from build123d import *

# Parameters (mm, degrees)
SKETCH1_W           = 25.4
SKETCH1_H           = 25.4
BOSS_EXTRUDE2_DEPTH = 254
SKETCH2_W           = 20.302766191
SKETCH2_H           = 19.05
CUT_EXTRUDE1_DEPTH  = 257.527425434
CUT_EXTRUDE2_DEPTH  = 257.527425434
SKETCH6_R           = 3.175
CUT_EXTRUDE5_DEPTH  = 257.527425553
SKETCH4_R           = 3.175
CUT_EXTRUDE6_DEPTH  = 257.527425553
SKETCH7_R           = 3.175
CUT_EXTRUDE7_DEPTH  = 257.527425553


with BuildPart() as part:
    # Sketch1 → Boss-Extrude2 (new body)
    with BuildSketch(Plane.XY):
        with Locations((12.7, 12.7)):
            Rectangle(SKETCH1_W, SKETCH1_H)
    extrude(amount=BOSS_EXTRUDE2_DEPTH)

    # Sketch2 → Cut-Extrude1 (cut, through all)
    with BuildSketch(Plane(origin=(0, 0, 0), x_dir=(-1, 0, 0), z_dir=(0, 0, -1))):
        with Locations((-13.326383096, 12.7)):
            Rectangle(SKETCH2_W, SKETCH2_H)
    extrude(amount=-CUT_EXTRUDE1_DEPTH, mode=Mode.SUBTRACT)

    # Sketch3 → Cut-Extrude2 (cut, through all)
    with BuildSketch(Plane(origin=(0, 25.4, 0), x_dir=(1, 0, 0), z_dir=(0, 1, 0))):
        with BuildLine():
            add(Edge.make_bspline(
                [(12.7, 0), (0, 0), (0, -30.465860076)],
                knots=[6.283185307, 6.283185307, 6.283185307, 7.853981634, 7.853981634, 7.853981634], degree=2, weights=[1, 0.707106781, 1]))
            Line((12.7, 0), (0, 0))
            Line((0, 0), (0, -30.465860076))
        make_face()
        with BuildLine():
            Line((25.4, 0), (12.7, 0))
            add(Edge.make_bspline(
                [(25.4, -30.465860076), (25.4, 0), (12.7, 0)],
                knots=[4.71238898, 4.71238898, 4.71238898, 6.283185307, 6.283185307, 6.283185307], degree=2, weights=[1, 0.707106781, 1]))
            Line((25.4, -30.465860076), (25.4, 0))
        make_face()
    extrude(amount=-CUT_EXTRUDE2_DEPTH, mode=Mode.SUBTRACT)

    # Sketch6 → Cut-Extrude5 (cut, through all)
    with BuildSketch(Plane(origin=(0, 25.4, 0), x_dir=(1, 0, 0), z_dir=(0, 1, 0))):
        with Locations(Location((12.7, -12.7, 0), (0, 0, 270))):
            Circle(SKETCH6_R)
    extrude(amount=-CUT_EXTRUDE5_DEPTH, mode=Mode.SUBTRACT)

    # Sketch4 → Cut-Extrude6 (cut, through all)
    with BuildSketch(Plane(origin=(0, 25.4, 0), x_dir=(1, 0, 0), z_dir=(0, 1, 0))):
        with Locations(Location((12.7, -101.6, 0), (0, 0, 270))):
            Circle(SKETCH4_R)
    extrude(amount=-CUT_EXTRUDE6_DEPTH, mode=Mode.SUBTRACT)

    # Sketch7 → Cut-Extrude7 (cut, through all)
    with BuildSketch(Plane(origin=(0, 25.4, 0), x_dir=(1, 0, 0), z_dir=(0, 1, 0))):
        with Locations(Location((12.7, -241.3, 0), (0, 0, 270))):
            Circle(SKETCH7_R)
    extrude(amount=-CUT_EXTRUDE7_DEPTH, mode=Mode.SUBTRACT)


solid = part.part
Geometry check sheet. Reference: the model listing, model coordinates, mm. A direction names the side the tool comes from. Give positions to 0.01 mm unless a question says otherwise; leave off trailing zeros. Loops run counter-clockwise (first coordinate to the right, second up) from the corner with the lowest first, then second, coordinate; pieces in that order, holes last. Notation, with made-up numbers: (22.5, -32.5) -> (63.5, -32.5) arc R15 ccw to (63.5, -12.5) -> close; hole circle Ø2 at (55, 6.25). An arc over 180 degrees is marked (long way). Answer in a Markdown table with one row per item. Add a question column.
1) Cross-section at B-B on z = 208.5. Record the boundary of the cut face in (x, y) (3 decimals), and give its area (3 significant figures).
2) Cross-section at A-A on z = 241.3. Record the boundary of the cut face in (x, y) (3 decimals).
3) Material ranges on probe 1 along Y at (x, z) = (21.25, 178) (3 decimals); probe 2 along X at (y, z) = (11, 57) (3 decimals); probe 3 along X at (y, z) = (24.5, 101.6) (3 decimals), recorded low to high. Write a range as from..to.
4) Cross-section at C-C on z = 101. Record the boundary of the cut face in (x, y) (3 decimals), and give its area (3 significant figures).
5) Set-up check for faces 1 (the face through (3.175, 13, 130)), 2 (the face through (10.77, 1.61, 10.18)): record each of +Z, -Z, +X, -X, +Y, -Y from which the full face is reachable in a straight line by a thin tool's end or side.
6) Draft check along X on faces 3 (the face through (13, 25.4, 125)), 4 (the face through (23.478, 13, 132)), 5 (the face through (25.4, 13, 141)). Enter one of: pulls with the +X half, pulls with the -X half, needs draft (parallel to the pull), parting line crosses it, or undercut.
7) Gauge pin test, flat end, axial feed: P1, Ø5, axis at x = 12.7, z = 12.7, coming from the -Y side. Record the tip position at first contact, or that the pin passes through.
Outcome:
| question | item | result |
|---|---|---|
| 1 | outline | (0, 0) -> (25.4, 0) -> (25.4, 25.4) -> (0, 25.4) -> close; hole (3.175, 3.175) -> (23.478, 3.175) -> (23.478, 22.225) -> (3.175, 22.225) -> close |
| 1 | area | 258 mm^2 |
| 2 | outline | (0, 0) -> (9.525, 0) -> (9.525, 3.175) -> (3.175, 3.175) -> (3.175, 22.225) -> (9.525, 22.225) -> (9.525, 25.4) -> (0, 25.4) -> close; (15.875, 0) -> (25.4, 0) -> (25.4, 25.4) -> (15.875, 25.4) -> (15.875, 22.225) -> (23.478, 22.225) -> (23.478, 3.175) -> (15.875, 3.175) -> close |
| 3 | probe 1 | y = 0..3.175, 22.225..25.4 |
| 3 | probe 2 | x = 0..3.175, 23.478..25.4 |
| 3 | probe 3 | x = 0..9.525, 15.875..25.4 |
| 4 | outline | (0, 0) -> (9.582, 0) -> (9.582, 3.175) -> (3.175, 3.175) -> (3.175, 22.225) -> (9.582, 22.225) -> (9.582, 25.4) -> (0, 25.4) -> close; (15.818, 0) -> (25.4, 0) -> (25.4, 25.4) -> (15.818, 25.4) -> (15.818, 22.225) -> (23.478, 22.225) -> (23.478, 3.175) -> (15.818, 3.175) -> close |
| 4 | area | 219 mm^2 |
| 5 | face 1 | +Z, -Z |
| 5 | face 2 | +Y, -Y |
| 6 | face 3 | needs draft |
| 6 | face 4 | undercut |
| 6 | face 5 | pulls with the +X half |
| 7 | P1 | passes through |
